from build123d import *

# Parameters (mm, degrees)
SKETCH1_R           = 100
SKETCH1_R_2         = 28
SKETCH1_R_3         = 10.15
BOSS_EXTRUDE1_DEPTH = 25


with BuildPart() as part:
    # Sketch1 → Boss-Extrude1 (new body)
    with BuildSketch(Plane(origin=(0, 0, 0), x_dir=(1, 0, 0), z_dir=(0, 1, 0))):
        Circle(SKETCH1_R)
        Circle(SKETCH1_R_2, mode=Mode.SUBTRACT)
        with Locations((0, 75)):
            Circle(SKETCH1_R_3, mode=Mode.SUBTRACT)
        with Locations((64.951905284, -37.5)):
            Circle(SKETCH1_R_3, mode=Mode.SUBTRACT)
        with Locations((-64.951905284, -37.5)):
            Circle(SKETCH1_R_3, mode=Mode.SUBTRACT)
    extrude(amount=BOSS_EXTRUDE1_DEPTH)


solid = part.part
Geometry: final body of the model. Coordinates: model frame, mm. Round coordinates to 2 decimals unless told otherwise and drop trailing zeros. Loops run counter-clockwise (first coordinate to the right, second up) from the corner with the lowest first, then second, coordinate; pieces in that order, holes last.
Q1. Section A-A on x = 0. Return loops of the section in (y, z), plus the area to 3 significant figures.
Q2. Material intervals for L1, parallel to Z at x = 0, y = 14; L2, parallel to X at y = 22.5, z = 31; L3, parallel to X at y = 8.75, z = 37.5, sorted ascending.
Q3. Section B-B on z = 0. Return loops of the section in (x, y).
Q4. Section C-C on z = 33. Return loops of the section in (x, y).
Q5. Pull-direction query (Z, two-part tool) for faces 1 (the flat face through (21, 25, 21)), 2 (the cylindrical face through (95.38, 12.32, -30.04)), 3 (the cylindrical face through (25.865, 12.325, 10.724)); classes: released by +Z, released by -Z, zero draft, split by the parting line, or undercut.
Q6. Pin query (flat end, axial travel): P1, Ø8, axis at y = 21, z = -71, coming from the -X side; P2, Ø2, axis at x = 53.5, y = 14, coming from the +Z side; P3, Ø6, axis at x = 43, y = 21.5, coming from the +Z side. Return the tip coordinate at first contact, or that it passes through.
Q7. Section D-D on y = 9.75. Return loops of the section in (x, z).
Evaluation:
1. outline: (0, -100) - (25, -100) - (25, -85.15) - (0, -85.15) - close; (0, -64.85) - (25, -64.85) - (25, -28) - (0, -28) - close; (0, 28) - (25, 28) - (25, 100) - (0, 100) - close
1. area: 3,090 mm2
2. L1: z = -100 to -85.15, -64.85 to -28, 28 to 100
2. L2: x = -95.07 to -72.75, -57.16 to 57.16, 72.75 to 95.07
2. L3: x = -92.7 to -75.1, -54.8 to 54.8, 75.1 to 92.7
3. outline: (-100, 0) - (-28, 0) - (-28, 25) - (-100, 25) - close; (28, 0) - (100, 0) - (100, 25) - (28, 25) - close
4. outline: (-94.4, 0) - (-74.05, 0) - (-74.05, 25) - (-94.4, 25) - close; (-55.85, 0) - (55.85, 0) - (55.85, 25) - (-55.85, 25) - close; (74.05, 0) - (94.4, 0) - (94.4, 25) - (74.05, 25) - close
5. face 1: zero draft
5. face 2: split by the parting line
5. face 3: undercut
6. P1: stops at x = -74.24
6. P2: stops at z = 85.11
6. P3: stops at z = 91.65
7. outline: circle Ø200 at (0, 0); hole circle Ø20.3 at (-64.95, 37.5); hole circle Ø56 at (0, 0); hole circle Ø20.3 at (0, -75); hole circle Ø20.3 at (64.95, 37.5)
